For this review, take the finished solid that the model builds, in its own axes (mm). Face numbers are marked on the shaded views. A direction names the side the tool comes from. Round coordinates to 2 decimals unless told otherwise and drop trailing zeros. Write each loop counter-clockwise with the first axis right and the second up, starting at its lowest first coordinate (ties: lowest second). Pieces come first, ordered by that corner, then holes. Notation, with made-up numbers: M -38,-35 L -30,-35 A18 ccw -30,0 Z; hole C 76,56 d9. An arc over 180 degrees is marked long. Answer in a Markdown table with one row per item.
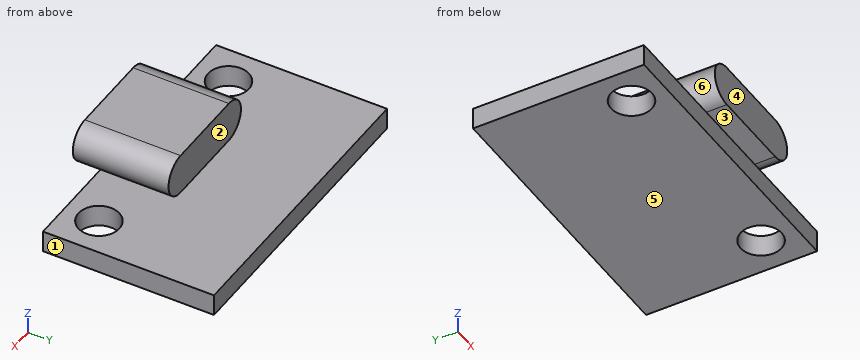
Autodesk Fusion 360 part; units mm, degrees
sketch "Skizze1" plane through (0, 0, 0) normal (0, 0, 1) x (1, 0, 0)
  line L0 (0, 0) -> (-21.5, 0)
  line L1 (-21.5, 0) -> (-21.5, 12.5)
  line L2 (-21.5, 12.5) -> (0, 12.5)
  line L3 (0, 12.5) -> (0, 0)
  circle A0 centre (-18.8, 2.5) radius 1.5
  circle A1 centre (-2.7, 2.5) radius 1.5
  line L4 (-21.5, 11.23) -> (0, 11.23) construction
  line L5 (-10.75, 12.5) -> (-10.75, 0) construction
  point P0 (-10.75, 11.23)
  dimension "d1" = 21.5
  dimension "d2" = 12.5
  dimension "d3" = 3
  dimension "d4" = 2.7
  dimension "d5" = 2.7
  dimension "d6" = 2.5
  dimension "d7" = 2.5
  dimension "d8" = 1.27
extrude "Extrusion1" add sketch "Skizze1" along normal blind 1.6
sketch "Skizze2" plane through (0, 0, 0) normal (0, -1, 0) x (1, 0, 0)
  line L0 (-21.5, 0) -> (0, 0)
  line L1 (0, 0) -> (0, 1.6)
  line L2 (0, 1.6) -> (-21.5, 1.6)
  line L3 (-21.5, 1.6) -> (-21.5, 0)
  line L4 (-10.75, 0) -> (-10.75, 13.6465) construction
  line L5 (-13.75, 4.6) -> (-7.75, 4.6)
  line L6 (-7.75, 1.6) -> (-13.75, 1.6)
  arc A0 (-13.75, 4.6) -> (-13.75, 1.6) centre (-13.75, 3.1) ccw
  arc A1 (-7.75, 1.6) -> (-7.75, 4.6) centre (-7.75, 3.1) ccw
  point P0 (-10.75, 1.6)
  dimension "d11" = 1.5
  dimension "d12" = 6
extrude "Extrusion2" add sketch "Skizze2" along normal blind 1.5 and the other way blind 5.5 contours L2 L5 L6 A0 A1
sketch "Skizze3" plane through (0, 0, 1.6) normal (0, 0, 1) x (-1, 0, 0)
  line L0 (7.75, -5.5) -> (7.75, 0)
  line L1 (7.75, 0) -> (0, 0)
  line L2 (0, 0) -> (0, -12.5)
  line L3 (0, -12.5) -> (21.5, -12.5)
  line L4 (21.5, -12.5) -> (21.5, 0)
  line L5 (21.5, 0) -> (13.75, 0)
  line L6 (13.75, 0) -> (13.75, -5.5)
  line L7 (13.75, -5.5) -> (7.75, -5.5)
  circle A0 centre (2.7, -2.5) radius 1.5
  circle A1 centre (18.8, -2.5) radius 1.5
  point P0 (10.75, -11.23)
  point P1 (10.75, -11.23)
ref_plane "Arbeitsebene1" through (0, 0, 5.1) normal (0, 0, 1) x (1, 0, 0)
sketch "Skizze4" plane through (0, 0, 5.1) normal (0, 0, 1) x (1, 0, 0)
  point P0 (-10.75, 11.23)
  point P1 (-10.75, 11.23)
equation "d4 = 1.2 mm + 1.5 mm"
equation "d5 = d4"
equation "d7 = d6"
equation "d8 = ( 2.54 / 2 ) * 1 mm"
equation "d12 = 9 mm - 3 mm"
equation "d15 = 7 mm - 1.5 mm"
equation "d17 = 1.6 mm + 3.5 mm"
Q1. Mouldability with a two-part tool opening along Z and no side actions: class the marked faces 4, 5 and 6 as +Z half, -Z half, draft (parallel to the pull), parting line (faces both ways), or undercut.
Found:
| item | result |
|---|---|
| face 4 | draft |
| face 5 | -Z half |
| face 6 | undercut |
Q2. For probe 1 along Y at (x, z) = (-18.8, 0.8); probe 2 along Y at (x, z) = (-13.75, 3.7); probe 3 along Z at (x, y) = (-10.5, 7.25), list the stretches that pass through material, from the lowest coordinate up.
Found:
| item | result |
|---|---|
| probe 1 | 0 to 1, 4 to 12.5 |
| probe 2 | -1.5 to 5.5 |
| probe 3 | 0 to 1.6 |
Q3. Take a section at C-C (x = -13). State the section outline as (y, z) points, then the cut area to 3 significant figures.
Found:
| item | result |
|---|---|
| outline | M -1.5,1.6 L 0,1.6 L 0,0 L 12.5,0 L 12.5,1.6 L 5.5,1.6 L 5.5,4.6 L -1.5,4.6 Z |
| area | 41.0 mm² |
Q4. Machinability: for the marked faces 1, 2 and 3, which of the approach directions +Z, -Z, +X, -X, +Y, -Y give a long, thin tool a straight path to every point of the face, cutting with its end or side? Answer none if there is none.
Found:
| item | result |
|---|---|
| face 1 | +Z, -Z, +X, +Y, -Y |
| face 2 | +Z, +X, -X, +Y |
| face 3 | -Z, +X, -X, -Y |
Q5. Insertion check: P1, Ø1.5, axis at x = -9.5, z = 4, coming from the +Y side; P2, Ø0.8, axis at x = -9.5, z = 0.5, coming from the -Y side; P3, Ø0.8, axis at x = -10.5, y = -0.5, coming from the -Z side; P4, Ø2, axis at y = 8, z = 3, coming from the -X side. Each pin has a flat end and moves straight along its axis. Give the tip position at first contact, or say it passes through.
Found:
| item | result |
|---|---|
| P1 | y = 5.5 |
| P2 | y = 0 |
| P3 | z = 1.6 |
| P4 | through |
Q6. Take a section at B-B (y = 2.5). State the section outline as (x, z) points, then the cut area to 3 significant figures.
Found:
| item | result |
|---|---|
| outline | M -21.5,0 L -20.3,0 L -20.3,1.6 L -21.5,1.6 Z; M -17.3,0 L -4.2,0 L -4.2,1.6 L -7.75,1.6 A1.5 ccw -7.75,4.6 L -13.75,4.6 A1.5 ccw -13.75,1.6 L -17.3,1.6 Z; M -1.2,0 L 0,0 L 0,1.6 L -1.2,1.6 Z |
| area | 49.9 mm² |
Q7. Take a section at D-D (y = 4.75). State the section outline as (x, z) points.
Found:
| item | result |
|---|---|
| outline | M -21.5,0 L 0,0 L 0,1.6 L -7.75,1.6 A1.5 ccw -7.75,4.6 L -13.75,4.6 A1.5 ccw -13.75,1.6 L -21.5,1.6 Z |
Q8. Take a section at A-A (x = -2.7). State the section outline as (y, z) points.
Found:
| item | result |
|---|---|
| outline | M 0,0 L 1,0 L 1,1.6 L 0,1.6 Z; M 4,0 L 12.5,0 L 12.5,1.6 L 4,1.6 Z |
